Could you check a few things on this model? Use its own coordinates, in mm. A direction names the side the tool comes from. Coordinates: 2 decimals unless noted, no trailing zeros. Write each loop counter-clockwise with the first axis right and the second up, starting at its lowest first coordinate (ties: lowest second). Pieces come first, ordered by that corner, then holes.
Item 1: Which directions (+Z, -Z, +X, -X, +Y, -Y) give clear straight access to the entire face, cutting with the end or side of a thin tool? Please do faces 1 (the cylindrical face through (33.672, -1.449, -13.825)), 2 (the cylindrical face through (33.672, -11.251, -13.825)), 3 (the flat face through (-17.164, -6.261, 21.774)).
Item 2: Thinking about a two-plate mould opening in X: for faces 4 (the flat face through (-13, 0, 13)), 5 (the cylindrical face through (-41.065, -1.449, 62.191)), 6 (the cylindrical face through (-14.96, -11.25, 44.47)), 7 (the cylindrical face through (-14.086, -6.332, -26.602)), which applies, +X half, -X half, draft (parallel to the pull), parting line (faces both ways), or undercut?
Item 3: If I drill on probe 1 along Z at (x, y) = (-11.5, -5.25); probe 2 along Z at (x, y) = (-3.5, -1.25); probe 3 along Z at (x, y) = (-26, -11.25), over which ranges is the centre line in solid material (lowest first)?
Item 4: For P1, Ø6, axis at y = -10.5, z = 32.5, coming from the -X side; P2, Ø6, axis at y = -8.5, z = 35, coming from the +X side; P3, Ø6, axis at y = -4.5, z = -18.5, coming from the -X side, each with a flat end and sliding along its axis, tell me the tip position at first contact or that it passes through.
Item 5: I want a section at A-A on y = -10.25. Please give me the cut outline in (x, z), then the cut area to 3 significant figures.
from build123d import *

# Parameters (mm, degrees)
F0_R     = 21.014231477
F1_DEPTH = 12.7
F2_F1_R  = 5.08
F2_F2_R  = 5.08


with BuildPart() as f1:
    # F0 (on Front) → F1 (new body)
    with BuildSketch(Plane.XZ):
        Polygon((-51.5739838451, 57.903360525), (-29.9211297043, 5.0337655893), (2.754318782, 23.7208167973), (-31.8911919502, 69.2358331578), align=None)
        Polygon((-32.4213020707, 59.6586255942), (-10.1648603382, 25.7348876013), (-24.3627145166, 17.7003582495), (-40.2510521891, 55.227790036), align=None, mode=Mode.SUBTRACT)
        Polygon((-29.9211297043, 5.0337655893), (-30.0753928796, -32.6075284839), (2.4457924315, -51.5617713492), (35.1212409178, -32.8747201412), (35.2755040931, 4.766573932), (2.754318782, 23.7208167973), align=None)
        with Locations((2.5902532507, -13.814676553)):
            Circle(F0_R, mode=Mode.SUBTRACT)
    extrude(amount=F1_DEPTH)

    # F2: fillet of radius 5.08 on 22 edges, made by hand

    # F2_f1
    f2_f1_edges = [f1.edges().sort_by_distance(p)[0] for p in [
        (-29.9211297043, -6.35, 5.0337655893),
        (2.754318782, -6.35, 23.7208167973),
    ]]
    fillet(f2_f1_edges, radius=F2_F1_R)

    # F2_f2
    f2_f2_edges = [f1.edges().sort_by_distance(p)[0] for p in [
        (-18.4239782263, -12.7, -13.814676553),
        (-30.0753928796, -6.35, -32.6075284839),
        (-30.0003324711, 0, -14.2922636402),
        (-30.0003324711, -12.7, -14.2922636402),
        (2.4457924315, -6.35, -51.5617713492),
        (-13.8148002241, 0, -42.0846499165),
        (-13.8148002241, -12.7, -42.0846499165),
        (35.1212409178, -6.35, -32.8747201412),
        (18.7835166747, 0, -42.2182457452),
        (18.7835166747, -12.7, -42.2182457452),
        (35.2755040931, -6.35, 4.766573932),
        (35.1983725055, 0, -14.0540731046),
        (35.1983725055, -12.7, -14.0540731046),
        (19.4511663483, 0, 13.9894339824),
        (19.4511663483, -12.7, 13.9894339824),
        (-31.8911919502, -6.35, 69.2358331578),
        (-51.5739838451, -6.35, 57.903360525),
        (-41.7325878977, 0, 63.5695968414),
        (-41.7325878977, -12.7, 63.5695968414),
        (-18.4239782263, 0, -13.814676553),
        (2.8201605652, -12.7, 23.7952939078),
        (2.8201605652, 0, 23.7952939078),
        (-30.0188752401, -12.7, 5.0147331632),
        (-30.0188752401, 0, 5.0147331632),
    ]]
    fillet(f2_f2_edges, radius=F2_F2_R)


solid = f1.part
Response values:
1. face 1: -Z, +X, +Y
1. face 2: -Z, +X, -Y
1. face 3: +Y, -Y
2. face 4: draft
2. face 5: -X half
2. face 6: +X half
2. face 7: undercut
3. probe 1: z = -43.43 to -29.41, 1.78 to 24.98, 27.77 to 42.45
3. probe 2: z = -46.08 to -35.74, 8.11 to 29.06
3. probe 3: z = -33.22 to 21.57, 49.87 to 58.98
4. P1: stops at x = -42.03
4. P2: stops at x = -3.6
4. P3: stops at x = -30.03
5. outline: (-49.21, 54.07) - (-29.63, 6.25) arc R5.81 cw to (-29.19, 4.02) - (-29.33, -29.68) arc R4.35 ccw to (-27.17, -33.45) - (0.28, -49.45) arc R4.35 ccw to (4.63, -49.47) - (32.21, -33.69) arc R4.35 ccw to (34.4, -29.94) - (34.53, 1.84) arc R4.35 ccw to (32.37, 5.61) - (3.26, 22.58) arc R5.81 cw to (1.56, 24.08) - (-29.77, 65.24) arc R4.35 ccw to (-35.4, 66.37) - (-47.36, 59.48) arc R4.35 ccw to start; hole (-40.25, 55.23) - (-24.36, 17.7) - (-10.16, 25.73) - (-32.42, 59.66) - close; hole circle Ø43.5 at (2.59, -13.81)
5. area: 3,150 mm2
